from build123d import *

# Parameters (mm, degrees)
F1_DEPTH = 46
F2_DEPTH = 46
F4_DEPTH = 25


with BuildPart() as f1:
    # F0 (on Front) → F1 (new body)
    with BuildSketch(Plane.XZ):
        with BuildLine():
            Line((-16, 16), (-16, 0))
            ThreePointArc((-16, 0), (0, -16), (16, 0))
            Line((16, 0), (134, 0))
            Line((134, 0), (134, 16))
            Line((134, 16), (-16, 16))
        make_face()
    extrude(amount=F1_DEPTH)

    # F0 (on Front) → F2 (join)
    with BuildSketch(Plane.XZ):
        with BuildLine():
            Line((-16, 16), (-16, 0))
            ThreePointArc((-16, 0), (0, -16), (16, 0))
            Line((16, 0), (134, 0))
            Line((134, 0), (134, 16))
            Line((134, 16), (-16, 16))
        make_face()
    extrude(amount=F2_DEPTH)

    # F3 (on face) → F4 (cut)
    with BuildSketch(Plane.XY.offset(16)):
        Polygon((134, -36.245503), (74, -46), (134, -46), align=None)
        Polygon((134, 0), (74, 0), (134, -5.8145), align=None)
    extrude(amount=-F4_DEPTH, mode=Mode.SUBTRACT)


solid = f1.part
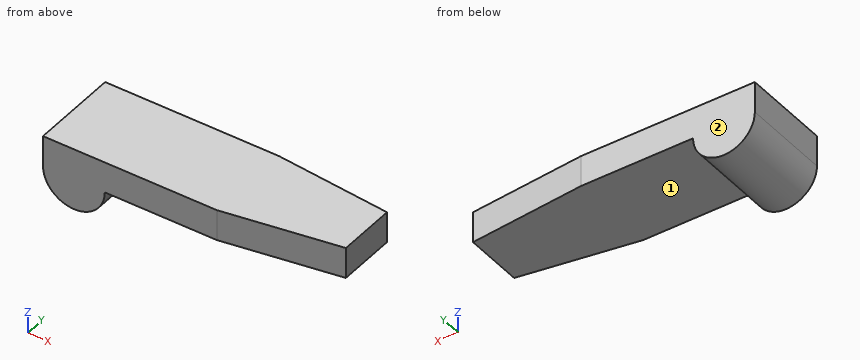
Geometry check sheet. Reference: the model listing, model coordinates, mm. Face numbers are marked on the shaded views. A direction names the side the tool comes from. Give positions to 0.01 mm unless a question says otherwise; leave off trailing zeros. Loops run counter-clockwise (first coordinate to the right, second up) from the corner with the lowest first, then second, coordinate; pieces in that order, holes last.
(1) Depth check by flat-ended pin: pin 1 Ø14 at (x, y) = (80, -29.5) entering from -Z; pin 2 Ø3 at (y, z) = (-37, -2.5) entering from -X; pin 3 Ø5 at (y, z) = (-15.5, -3.5) entering from +X. Enter the tip coordinate at first touch or a pass-through.
From the geometry:
pin 1: stops at z = 0
pin 2: stops at x = -15.97
pin 3: stops at x = 15.97
(2) Thickness scan on L1, parallel to Z at x = 102.5, y = -31; L2, parallel to Z at x = 3, y = -5.5; L3, parallel to X at y = -10, z = -6. Record the ranges inside material, lowest first.
From the geometry:
L1: z = 0 to 16
L2: z = -15.72 to 16
L3: x = -14.83 to 14.83
(3) Section check C-C on z = 12. Record the cut outline in (x, y).
From the geometry:
outline: (-16, -46) - (74, -46) - (134, -36.25) - (134, -5.81) - (74, 0) - (-16, 0) - close
(4) Section check D-D on z = -5. Record the cut outline in (x, y), then the cut area to 3 significant figures.
From the geometry:
outline: (-15.2, -46) - (15.2, -46) - (15.2, 0) - (-15.2, 0) - close
area: 1,400 mm2
(5) Section check B-B on x = 28.5. Record the cut outline in (y, z), then the cut area to 3 significant figures.
From the geometry:
outline: (-46, 0) - (0, 0) - (0, 16) - (-46, 16) - close
area: 736 mm2
(6) Set-up check for the marked faces 1 and 2: record each of +Z, -Z, +X, -X, +Y, -Y from which the full face is reachable in a straight line by a thin tool's end or side.
From the geometry:
face 1: -Z, +X, +Y, -Y
face 2: +Z, -Z, +X, -X, +Y
(7) Section check A-A on y = -11. Record the cut outline in (x, z), then the cut area to 3 significant figures.
From the geometry:
outline: (-16, 0) arc R16 ccw to (16, 0) - (134, 0) - (134, 16) - (-16, 16) - close
area: 2,800 mm2
